from build123d import *

# Parameters (mm, degrees)
BOSS_EXTRUDE4_DEPTH = 25.4
CUT_EXTRUDE1_REACH  = 35.668
SKETCH7_R           = 3.175
SKETCH9_W           = 14.069203901
SKETCH9_H           = 9.525
CUT_EXTRUDE2_DEPTH  = 25.4
SKETCH10_W          = 12.7
SKETCH10_H          = 9.525
BOSS_EXTRUDE5_DEPTH = 12.7
SKETCH11_R          = 1.5875
CUT_EXTRUDE3_DEPTH  = 12.7
SKETCH13_W          = 13.214088126
SKETCH13_H          = 21.166666667
CUT_EXTRUDE5_DEPTH  = 9.525
SKETCH14_W          = 12.7
SKETCH14_H          = 9.525
BOSS_EXTRUDE6_DEPTH = 12.7
CUT_EXTRUDE7_DEPTH  = 12.7
BOSS_EXTRUDE7_DEPTH = 9.525
SKETCH17_R          = 3.175
BOSS_EXTRUDE8_DEPTH = 15.875
SKETCH18_R          = 3.571875
CUT_EXTRUDE8_DEPTH  = 15.875
SKETCH19_R          = 1.587499998
CUT_EXTRUDE9_DEPTH  = 15.875
SKETCH20_R          = 1.587499998
BOSS_EXTRUDE9_DEPTH = 3.81
SKETCH21_R          = 3.429
CUT_EXTRUDE10_DEPTH = 12.7


with BuildPart() as part:
    # Sketch6 → Boss-Extrude4 (new body)
    with BuildSketch(Plane(origin=(0, 0, 0), x_dir=(1, 0, 0), z_dir=(0, 1, 0))):
        with BuildLine():
            Line((-6.35, -21.166666667), (6.35, -21.166666667))
            Line((6.35, -21.166666667), (6.35, 10.583333333))
            ThreePointArc((6.35, 10.583333333), (0, 16.933333333), (-6.35, 10.583333333))
            Line((-6.35, 10.583333333), (-6.35, -21.166666667))
        make_face()
    extrude(amount=BOSS_EXTRUDE4_DEPTH)

    # Sketch7 → Cut-Extrude1 (cut, up to next)
    with BuildSketch(Plane.XZ, mode=Mode.PRIVATE) as cut_extrude1_sk1:
        with Locations(Location((0, -10.583333333, 0), (0, 0, 270))):
            Circle(SKETCH7_R)
    cut_extrude1_tool1 = extrude(cut_extrude1_sk1.sketch, amount=-CUT_EXTRUDE1_REACH, mode=Mode.PRIVATE) & part.part
    add(cut_extrude1_tool1.solids().sort_by_distance((0, 0, -10.583333))[0], mode=Mode.SUBTRACT)

    # Sketch9 → Cut-Extrude2 (cut)
    with BuildSketch(Plane.XY.offset(-16.933333333)):
        with Locations((0.122145241, 4.7625)):
            Rectangle(SKETCH9_W, SKETCH9_H)
    extrude(amount=CUT_EXTRUDE2_DEPTH, mode=Mode.SUBTRACT)

    # Sketch10 → Boss-Extrude5 (add)
    with BuildSketch(Plane(origin=(6.35, 0, 0), x_dir=(0, 0, -1), z_dir=(1, 0, 0))):
        with Locations((-14.816666667, 4.7625)):
            Rectangle(SKETCH10_W, SKETCH10_H)
    extrude(amount=BOSS_EXTRUDE5_DEPTH)

    # Sketch11 → Cut-Extrude3 (cut)
    with BuildSketch(Plane(origin=(0, 9.525, 0), x_dir=(1, 0, 0), z_dir=(0, 1, 0))):
        with BuildLine():
            ThreePointArc((15.875, -8.466666667), (15.927897388, -8.467107348), (15.980780092, -8.468429271))
            ThreePointArc((15.980780092, -8.468429271), (18.157156523, -9.434318347), (19.05, -11.641666667))
            Line((19.05, -11.641666667), (19.05, -8.466666667))
            Line((19.05, -8.466666667), (15.875, -8.466666667))
        make_face()
        with BuildLine():
            Line((12.847839644, -12.599228768), (6.35, -21.166666667))
            Line((6.35, -21.166666667), (19.05, -21.166666667))
            Line((19.05, -21.166666667), (19.05, -11.641666667))
            ThreePointArc((19.05, -11.641666667), (16.359453749, -14.779489091), (12.847839644, -12.599228768))
        make_face()
        with Locations(Location((15.875, -11.641666667, 0), (0, 0, 270))):
            Circle(SKETCH11_R)
    extrude(amount=-CUT_EXTRUDE3_DEPTH, mode=Mode.SUBTRACT)

    # Sketch13 → Cut-Extrude5 (cut)
    with BuildSketch(Plane(origin=(0, 9.525, 0), x_dir=(1, 0, 0), z_dir=(0, 1, 0))):
        with Locations((12.957044063, -10.583333334)):
            Rectangle(SKETCH13_W, SKETCH13_H)
    extrude(amount=-CUT_EXTRUDE5_DEPTH, mode=Mode.SUBTRACT)

    # Sketch14 → Boss-Extrude6 (add)
    with BuildSketch(Plane.ZY.offset(6.35)):
        with Locations((14.816666667, 4.7625)):
            Rectangle(SKETCH14_W, SKETCH14_H)
    extrude(amount=BOSS_EXTRUDE6_DEPTH)

    # Sketch15 → Cut-Extrude7 (cut)
    with BuildSketch(Plane(origin=(0, 9.525, 0), x_dir=(1, 0, 0), z_dir=(0, 1, 0))):
        Polygon((-6.35, -8.466666667), (-14.506048031, -8.466666667), (-19.05, -8.466666667), (-19.05, -21.166666667), (-6.35, -21.166666667), align=None)
    extrude(amount=-CUT_EXTRUDE7_DEPTH, mode=Mode.SUBTRACT)

    # Sketch16 → Boss-Extrude7 (add)
    with BuildSketch(Plane(origin=(0, 9.525, 0), x_dir=(1, 0, 0), z_dir=(0, 1, 0))):
        Polygon((-17.681048031, -21.166666667), (-6.35, -21.166666667), (-6.35, -8.466666667), (-13.303781858, -8.466666667), (-17.681048031, -8.466666667), (-17.681048031, -11.641666667), align=None)
    extrude(amount=-BOSS_EXTRUDE7_DEPTH)

    # Sketch17 → Boss-Extrude8 (add)
    with BuildSketch(Plane.XZ.offset(-9.525)):
        with Locations((0, -10.583333333)):
            Circle(SKETCH17_R)
    extrude(amount=-BOSS_EXTRUDE8_DEPTH)

    # Sketch18 → Cut-Extrude8 (cut)
    with BuildSketch(Plane.XZ.offset(-9.525)):
        with Locations((0, -10.583333333)):
            Circle(SKETCH18_R)
    extrude(amount=-CUT_EXTRUDE8_DEPTH, mode=Mode.SUBTRACT)

    # Sketch19 → Cut-Extrude9 (cut)
    with BuildSketch(Plane(origin=(0, 9.525, 0), x_dir=(1, 0, 0), z_dir=(0, 1, 0))):
        with Locations(Location((-14.50604803, -11.641666664, 0), (0, 0, 270))):
            Circle(SKETCH19_R)
        with BuildLine():
            Line((-17.681048031, -8.466666667), (-14.50604803, -8.466666667))
            Line((-14.50604803, -8.466666667), (-14.50604803, -8.479366664))
            ThreePointArc((-14.50604803, -8.479366664), (-17.523471535, -10.695465482), (-16.311752542, -14.237735328))
            Line((-16.311752542, -14.237735328), (-6.35, -21.166666667))
            Line((-6.35, -21.166666667), (-17.681048031, -21.166666667))
            Line((-17.681048031, -21.166666667), (-17.681048031, -8.466666667))
        make_face()
    extrude(amount=-CUT_EXTRUDE9_DEPTH, mode=Mode.SUBTRACT)

    # Sketch20 → Boss-Extrude9 (add)
    with BuildSketch(Plane.XZ):
        with BuildLine():
            Line((-6.35, 21.166666667), (6.35, 21.166666667))
            Line((6.35, 21.166666667), (6.35, 8.466666667))
            Line((6.35, 8.466666667), (-14.50604803, 8.479366664))
            ThreePointArc((-14.50604803, 8.479366664), (-17.523471535, 10.695465482), (-16.311752542, 14.237735328))
            Line((-16.311752542, 14.237735328), (-6.35, 21.166666667))
        make_face()
        with Locations(Location((-14.50604803, 11.641666664, 0), (0, 0, 90))):
            Circle(SKETCH20_R, mode=Mode.SUBTRACT)
    extrude(amount=BOSS_EXTRUDE9_DEPTH)

    # Sketch21 → Cut-Extrude10 (cut)
    with BuildSketch(Plane.XY.offset(21.166666667)):
        with Locations((0, 2.54)):
            Circle(SKETCH21_R)
    extrude(amount=-CUT_EXTRUDE10_DEPTH, mode=Mode.SUBTRACT)


solid = part.part
Model file for the job. Use its own axes, mm. A direction names the side the tool comes from. Round coordinates to 2 decimals unless told otherwise and drop trailing zeros. Loops run counter-clockwise (first coordinate to the right, second up) from the corner with the lowest first, then second, coordinate; pieces in that order, holes last.
1. Drop flat-ended pins along their axis: P1, Ø1.5, axis at x = 0, z = 1.5, coming from the -Y side (3 decimals); P2, Ø8, axis at y = 18.5, z = 0, coming from the -X side; P3, Ø3, axis at x = -8.5, y = 7, coming from the -Z side. Give the stop position or say it passes through.
Check values:
P1: stops at y = 9.525
P2: stops at x = -6.35
P3: stops at z = 8.47
2. Band-saw the part on B-B, the plane x = 0. List the corners of the cut face in (y, z) (3 decimals).
Check values:
outline: (-3.81, 8.471) - (-0.889, 8.471) - (-0.889, 21.167) - (-3.81, 21.167) - close; (5.969, 8.467) - (9.525, 8.467) - (9.525, -7.011) - (25.4, -7.011) - (25.4, 21.167) - (5.969, 21.167) - close; (9.525, -16.933) - (25.4, -16.933) - (25.4, -14.155) - (9.525, -14.155) - close
3. Band-saw the part on C-C, the plane y = 19.25. List the corners of the cut face in (x, z).
Check values:
outline: (-6.35, -10.58) arc R6.35 ccw to (6.35, -10.58) - (6.35, 21.17) - (-6.35, 21.17) - close; hole circle Ø7.14 at (0, -10.58)
4. Tool access for faces 1 (the flat face through (0, 9.525, -1)), 2 (the flat face through (-3, -3.81, 15)), 3 (the flat face through (-11, 9.525, 13)): list every direction of +Z, -Z, +X, -X, +Y, -Y with a clear straight run to the whole face (end or side of a thin tool).
Check values:
face 1: -Z, +X, -X, -Y
face 2: +Z, -Z, +X, -X, -Y
face 3: +Z, -Z, -X, +Y
5. Mould opens along X. For faces 4 (the flat face through (6.35, 14, 9)), 5 (the cylindrical face through (3.27, 3.57, 14.91)), 6 (the cylindrical face through (-17.506, 2.951, 10.642)) say: +X half, -X half, draft (parallel to the pull), parting line (faces both ways), or undercut.
Check values:
face 4: +X half
face 5: undercut
face 6: -X half
6. Band-saw the part on D-D, the plane x = -15. List the corners of the cut face in (y, z) (3 decimals), and give its area (3 significant figures).
Check values:
outline: (-3.81, 8.518) - (9.525, 8.518) - (9.525, 10.133) - (-3.81, 10.133) - close; (-3.81, 13.15) - (9.525, 13.15) - (9.525, 15.15) - (-3.81, 15.15) - close
area: 48.2 mm2
7. Wall check: probe 1 along X at (y, z) = (20.5, 14); probe 2 along Y at (x, z) = (-3.5, -12.5) (3 decimals); probe 3 along Z at (x, y) = (4, 4.25). Give the ranges that are in metal, low to high.
Check values:
probe 1: x = -6.35 to 6.35
probe 2: y = 9.525 to 25.4
probe 3: z = 8.47 to 21.17
8. Band-saw the part on A-A, the plane y = 2.54. Count the separate pieces of the cut face and the enclosed holes in it, and give its area (3 significant figures).
Check values:
separate pieces: 2
enclosed holes: 1
area: 163 mm2
